CAD build for the part. Positions are in the model's coordinates, mm. Face numbers are marked on the shaded views. A direction names the side the tool comes from. Round coordinates to 2 decimals unless told otherwise and drop trailing zeros. Write each loop counter-clockwise with the first axis right and the second up, starting at its lowest first coordinate (ties: lowest second). Pieces come first, ordered by that corner, then holes. Notation, with made-up numbers: (10, 19.25) - (69, 19.25) arc R29 cw to (69, 49.25) - close; hole circle Ø1 at (-1, -33). An arc over 180 degrees is marked (long way). Answer in a Markdown table with one row per item.
```python
from build123d import *

# Parameters (mm, degrees)
SKETCH3_W                                       = 57.15
SKETCH3_H                                       = 50
BOSS_EXTRUDE1_DEPTH                             = 8
SKETCH3_3_R                                     = 1.5
SKETCH3_3_R_2                                   = 8
CUT_EXTRUDE2_DEPTH                              = 10
SKETCH4_R                                       = 18.5
CUT_EXTRUDE3_DEPTH                              = 4
BOSS_EXTRUDE2_DEPTH                             = 15
BOSS_EXTRUDE2_DEPTH_BACK                        = 23
SKETCH6_W                                       = 80
SKETCH6_H                                       = 5
CSK_FOR_M3_FLAT_HEAD_MACHINE_SCREW1_D           = 3.4
CSK_FOR_M3_FLAT_HEAD_MACHINE_SCREW1_CSINK_D     = 6.3
CSK_FOR_M3_FLAT_HEAD_MACHINE_SCREW1_CSINK_ANGLE = 90
BOSS_EXTRUDE4_DEPTH                             = 2.54


with BuildPart() as part:
    # Sketch3 → Boss-Extrude1 (new body)
    with BuildSketch(Plane.XY):
        with Locations((0, 25)):
            Rectangle(SKETCH3_W, SKETCH3_H)
    extrude(amount=BOSS_EXTRUDE1_DEPTH)

    # Sketch3_3 → Cut-Extrude2 (cut)
    with BuildSketch(Plane.XY):
        with Locations(Location((-7.75, 38.423393759, 0), (0, 0, 180))):
            Circle(SKETCH3_3_R)
        with Locations(Location((7.75, 38.423393759, 0), (0, 0, 180))):
            Circle(SKETCH3_3_R)
        with Locations(Location((-7.75, 11.576606241, 0), (0, 0, 180))):
            Circle(SKETCH3_3_R)
        with Locations(Location((7.75, 11.576606241, 0), (0, 0, 180))):
            Circle(SKETCH3_3_R)
        with Locations(Location((15.5, 25, 0), (0, 0, 180))):
            Circle(SKETCH3_3_R)
        with Locations(Location((6.062177825, 28.499999999, 0), (0, 0, 180))):
            Circle(SKETCH3_3_R_2)
    extrude(amount=CUT_EXTRUDE2_DEPTH, mode=Mode.SUBTRACT)

    # Sketch4 → Cut-Extrude3 (cut)
    with BuildSketch(Plane.XY.offset(8)):
        with Locations((0, 25)):
            Circle(SKETCH4_R)
    extrude(amount=-CUT_EXTRUDE3_DEPTH, mode=Mode.SUBTRACT)

    # Sketch6 → Boss-Extrude2 (add, two sides: drawn at the far end of the back side and taken through both)
    with BuildSketch(Plane.XY.offset(8).offset(-BOSS_EXTRUDE2_DEPTH_BACK)):
        with Locations((0, 2.5)):
            Rectangle(SKETCH6_W, SKETCH6_H)
    extrude(amount=BOSS_EXTRUDE2_DEPTH + BOSS_EXTRUDE2_DEPTH_BACK)

    # CSK for M3 Flat Head Machine Screw1 (through all)
    with Locations(Plane(origin=(0, 5, 0), x_dir=(1, 0, 0), z_dir=(0, 1, 0))):
        with Locations((-32.5, 7.5), (-32.5, -15.5), (32.5, -15.5), (32.5, 7.5)):
            CounterSinkHole(CSK_FOR_M3_FLAT_HEAD_MACHINE_SCREW1_D / 2, CSK_FOR_M3_FLAT_HEAD_MACHINE_SCREW1_CSINK_D / 2, counter_sink_angle=CSK_FOR_M3_FLAT_HEAD_MACHINE_SCREW1_CSINK_ANGLE)

    # Sketch13 → Boss-Extrude4 (add)
    with BuildSketch(Plane(origin=(0, 0, 0), x_dir=(-1, 0, 0), z_dir=(0, 0, -1))):
        with BuildLine():
            Line((20.564, 22.023), (12.944, 22.023))
            ThreePointArc((12.944, 22.023), (6.467, 28.5), (12.944, 34.977))
            Line((12.944, 34.977), (20.564, 34.977))
            ThreePointArc((20.564, 34.977), (27.041, 28.5), (20.564, 22.023))
        make_face()
        with BuildLine():
            Line((20.564, 23.293), (12.944, 23.293))
            ThreePointArc((12.944, 23.293), (7.737, 28.5), (12.944, 33.707))
            Line((12.944, 33.707), (20.564, 33.707))
            ThreePointArc((20.564, 33.707), (25.771, 28.5), (20.564, 23.293))
        make_face(mode=Mode.SUBTRACT)
    extrude(amount=BOSS_EXTRUDE4_DEPTH)


solid = part.part
```
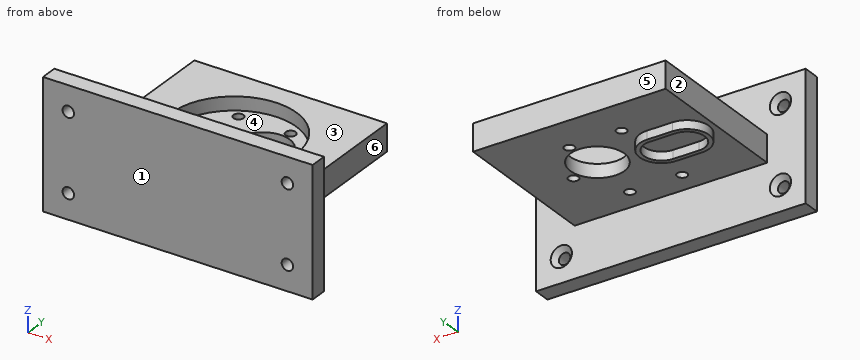
Q1. Pull direction X, two halves, no side cores. Call the marked faces 4, 5 and 6: released by +X, released by -X, zero draft, split by the parting line, or undercut.
Computed:
| item | result |
|---|---|
| face 4 | undercut |
| face 5 | zero draft |
| face 6 | released by +X |
Q2. Saw through at A-A on z = 15.5. List the corners of the cut face in (x, y).
Computed:
| item | result |
|---|---|
| outline | (-40, 0) - (-34.2, 0) - (-34.2, 3.55) - (-35.65, 5) - (-40, 5) - close; (-30.8, 0) - (30.8, 0) - (30.8, 3.55) - (29.35, 5) - (-29.35, 5) - (-30.8, 3.55) - close; (34.2, 0) - (40, 0) - (40, 5) - (35.65, 5) - (34.2, 3.55) - close |
Q3. Drill centre lines: line 1 (Y direction, x = -7.75, z = 2.95); line 2 (Z direction, x = 32.5, y = 1.25); line 3 (X direction, y = 0.8, z = -7.5). Where is each one in solid material? Low to high.
Computed:
| item | result |
|---|---|
| line 1 | y = 0 to 10.08, 13.08 to 36.92, 39.92 to 50 |
| line 2 | z = -15 to -9.2, -5.8 to 13.8, 17.2 to 23 |
| line 3 | x = -40 to -34.2, -30.8 to 30.8, 34.2 to 40 |
Q4. Saw through at D-D on x = 7.75. List the corners of the cut face in (y, z).
Computed:
| item | result |
|---|---|
| outline | (0, -15) - (5, -15) - (5, 0) - (10.08, 0) - (10.08, 4) - (8.2, 4) - (8.2, 8) - (5, 8) - (5, 23) - (0, 23) - close; (13.08, 0) - (20.68, 0) - (20.68, 4) - (13.08, 4) - close; (36.32, 0) - (36.92, 0) - (36.92, 4) - (36.32, 4) - close; (39.92, 0) - (50, 0) - (50, 8) - (41.8, 8) - (41.8, 4) - (39.92, 4) - close |
Q5. Saw through at C-C on x = 22. List the corners of the cut face in (y, z).
Computed:
| item | result |
|---|---|
| outline | (0, -15) - (5, -15) - (5, 0) - (50, 0) - (50, 8) - (5, 8) - (5, 23) - (0, 23) - close |
Q6. Flat gauge pins, fed straight in: pin 1 (6 mm diameter, centred on y = 35.5, z = -4, fed in from +X); pin 2 (1.3 mm diameter, centred on x = -18, z = -1.5, fed in from +Y); pin 3 (4 mm diameter, centred on y = 23, z = 2, fed in from -X) (3 decimals). Where does each tip first touch, or does it go through?
Computed:
| item | result |
|---|---|
| pin 1 | stops at x = -8.17 |
| pin 2 | stops at y = 34.98 |
| pin 3 | stops at x = -28.575 |
Q7. 3-axis set-ups, long thin cutter, end or side, ignore diameter. For the marked faces 1, 2 and 3: which of +Z, -Z, +X, -X, +Y, -Y reach the whole face in a straight line?
Computed:
| item | result |
|---|---|
| face 1 | +Z, -Z, +X, -X, -Y |
| face 2 | +Z, -Z, -X, +Y |
| face 3 | +Z, +X, -X, +Y |
Q8. Saw through at B-B on x = 32.5. List the corners of the cut face in (y, z), then the cut area to 3 significant figures.
Computed:
| item | result |
|---|---|
| outline | (0, -15) - (5, -15) - (5, -10.65) - (3.55, -9.2) - (0, -9.2) - close; (0, -5.8) - (3.55, -5.8) - (5, -4.35) - (5, 12.35) - (3.55, 13.8) - (0, 13.8) - close; (0, 17.2) - (3.55, 17.2) - (5, 18.65) - (5, 23) - (0, 23) - close |
| area | 152 mm2 |
